from build123d import *

# Parameters (mm, degrees)
SKETCH004_W  = 4
SKETCH004_H  = 60
PAD004_DEPTH = 7.5
PAD005_DEPTH = 30
SKETCH002_R  = 3
PAD006_DEPTH = 5
SKETCH003_R  = 2
PAD003_DEPTH = 40
PAD_DEPTH    = 7.5


with BuildPart() as pad004:
    # Sketch004 → Pad004 (new body, symmetric)
    with BuildSketch(Plane.XZ.offset(7.5)):
        with Locations((-0.160987, 0)):
            Rectangle(SKETCH004_W, SKETCH004_H)
    extrude(amount=PAD004_DEPTH, both=True)


with BuildPart() as pad005:
    # Sketch001 → Pad005 (new body)
    with BuildSketch(Plane(origin=(0, 0, 2), x_dir=(-1, 0, 0), z_dir=(0, 0, 1))):
        with BuildLine():
            ThreePointArc((-3.5, 3), (-6.5, 0), (-3.5, -3))
            Line((-3.5, -3), (3.5, -3))
            ThreePointArc((3.5, -3), (6.5, 0), (3.5, 3))
            Line((-3.5, 3), (3.5, 3))
        make_face()
    extrude(amount=PAD005_DEPTH)


with BuildPart() as pad006:
    # Sketch002 → Pad006 (new body, symmetric)
    with BuildSketch(Plane.XY.offset(2)):
        Circle(SKETCH002_R)
    extrude(amount=PAD006_DEPTH, both=True)


with BuildPart() as fusion:
    # Sketch003 → Pad003 (new body, symmetric)
    with BuildSketch(Plane.XY.offset(2)):
        Circle(SKETCH003_R)
    extrude(amount=PAD003_DEPTH, both=True)

    # Fusion: union Pad004, Pad005, Pad006
    add(pad004.part)
    add(pad005.part)
    add(pad006.part)


with BuildPart() as cut:
    # Sketch → Pad (new body, symmetric)
    with BuildSketch(Plane.XZ):
        Polygon((-8, 20), (-8, 0), (-5, 0), (-5, -5), (5, -5), (5, 0), (8, 0), (8, 20), align=None)
    extrude(amount=PAD_DEPTH, both=True)

    # Cut: cut Fusion
    add(fusion.part, mode=Mode.SUBTRACT)


solid = cut.part
Source: CAD feature listing. Evaluate the final solid. Frame: model axes, mm. A direction names the side the tool comes from. Give positions to 0.01 mm unless a question says otherwise; leave off trailing zeros. Write each loop counter-clockwise with the first axis right and the second up, starting at its lowest first coordinate (ties: lowest second). Pieces come first, ordered by that corner, then holes. Notation, with made-up numbers: M 85.25,-37 L 102.25,-37 A13 ccw 102.25,-29 Z; hole C 74,-32.75 d9. An arc over 180 degrees is marked long. Answer as a JSON object with one key per item and string values.
Q1. Mould query, pull axis Y, two halves, no side actions, for faces 5 (the face through (0, 7.5, 8)), 6 (the face through (-7, 0, 0)), 7 (the face through (3, -3, 11)), 8 (the face through (6.5, -0.1, 10.9)). Classes: +Y half, -Y half, draft (parallel to the pull), parting line (faces both ways), or undercut.
Geometry check:
{"face 5": "+Y half", "face 6": "draft", "face 7": "undercut", "face 8": "undercut"}
Q2. Cut plane C-C, the plane z = 11.25. Return the cut outline in (x, y), then the cut area to 3 significant figures.
Geometry check:
{"outline": "M -8,-7.5 L -2.16,-7.5 L -2.16,-3 L -3.5,-3 A3 cw -3.5,3 L 3.5,3 A3 cw 3.5,-3 L 1.84,-3 L 1.84,-7.5 L 8,-7.5 L 8,7.5 L -8,7.5 Z", "area": "152 mm^2"}
Q3. Cut plane A-A, the plane y = -5.5. Return the cut outline in (x, z), then the cut area to 3 significant figures.
Geometry check:
{"outline": "M -8,0 L -5,0 L -5,-5 L -2.16,-5 L -2.16,20 L -8,20 Z; M 1.84,-5 L 5,-5 L 5,0 L 8,0 L 8,20 L 1.84,20 Z", "area": "270 mm^2"}
Q4. Contact query for flat-ended pins moving along their axis: P1, Ø4.5, axis at x = 0, y = 0, coming from the +Z side; P2, Ø1.5, axis at x = 6, y = 0, coming from the -Z side; P3, Ø3, axis at x = 4, y = 0.5, coming from the +Z side. Output: stop coordinate, or through.
Geometry check:
{"P1": "stops at z = -3", "P2": "stops at z = 0", "P3": "stops at z = 2"}
Q5. Access query for faces 1 (the face through (-5, 0, -2)), 2 (the face through (-2.161, -5, 7)), 3 (the face through (0, 3, 11)), 4 (the face through (6, 0, 0)). Directions: +Z, -Z, +X, -X, +Y, -Y. A direction counts if a zero-diameter tool reaches every point of the face in a straight line with its end or side. Return the directions, or none.
Geometry check:
{"face 1": "-Z, -X, +Y, -Y", "face 2": "+Z, -Z, -Y", "face 3": "+Z", "face 4": "-Z, +X, +Y, -Y"}
Q6. Cut plane D-D, the plane y = 0.5. Return the cut outline in (x, z), then the cut area to 3 significant figures.
Geometry check:
{"outline": "M -8,0 L -5,0 L -5,-5 L -1.94,-5 L -1.94,-3 L -2.96,-3 L -2.96,2 L -6.46,2 L -6.46,20 L -8,20 Z; M 1.94,-5 L 5,-5 L 5,0 L 8,0 L 8,20 L 6.46,20 L 6.46,2 L 2.96,2 L 2.96,-3 L 1.94,-3 Z", "area": "100 mm^2"}
Q7. Ray query, line 1 along X through (y, z) = (0, 0.75); line 2 along X through (y, z) = (0, -0.9); line 3 along Y through (x, z) = (-3, 7). Return the intervals inside material, ascending.
Geometry check:
{"line 1": "x = -8 to -3, 3 to 8", "line 2": "x = -5 to -3, 3 to 5", "line 3": "y = -7.5 to -3, 3 to 7.5"}
Q8. Cut plane B-B, the plane y = 4.25. Return the cut outline in (x, z), then the cut area to 3 significant figures.
Geometry check:
{"outline": "M -8,0 L -5,0 L -5,-5 L 5,-5 L 5,0 L 8,0 L 8,20 L -8,20 Z", "area": "370 mm^2"}
